Model file for the job. Use its own axes, mm. A direction names the side the tool comes from. Coordinates: 2 decimals unless noted, no trailing zeros. Order: outer loops, then holes, each group sorted by start corner. A loop starts at its lowest first (then second) coordinate and runs counter-clockwise, first axis right, second up. Notation, with made-up numbers: (62, 3.5) -> (94, 3.5) arc R18 cw to (94, 30.5) -> close; hole circle Ø1 at (-1, 13). An arc over 180 degrees is marked (long way). Return JSON: item names as keys, results as strings. Group by question number.
1) Probe line 1 (Y direction, x = -23.5, z = 47); line 2 (X direction, y = -41, z = 18); line 3 (Z direction, x = -39, y = -30.5). List the from-to ranges inside material, lowest first.
2) Cut at A-A (z = 11). Write the cut outline in (x, y), and give its area (3 significant figures).
3) Flat gauge pins, fed straight in: pin 1 (8 mm diameter, centred on y = -40.5, z = 21.5, fed in from +X); pin 2 (1 mm diameter, centred on y = -41.5, z = 12.5, fed in from -X). Where does each tip first touch, or does it go through?
4) Cut at B-B (x = -24.5). Write the cut outline in (y, z).
5) Which spindle directions (+Z, -Z, +X, -X, +Y, -Y) get a long thin tool onto all of the face, cutting with end or side? Do faces 1 (the flat face through (-25.588, -38, 14)), 2 (the flat face through (-43.156, -38, 14)), 3 (the flat face through (-32, -19, 0)). Say none if no direction does.
6) Cut at C-C (y = -45). Write the cut outline in (x, z), and give its area (3 significant figures).
7) Cut at D-D (x = -28.5). Write the cut outline in (y, z), and give its area (3 significant figures).
from build123d import *

# Parameters (mm, degrees)
F0_W     = 39.718569
F0_H     = 51.366802
F1_DEPTH = 25.4
F3_DEPTH = 25.4


with BuildPart() as f1:
    # F0 (on Front) → F1 (new body)
    with BuildSketch(Plane.XZ):
        with Locations((-31.316563, 25.683401)):
            Rectangle(F0_W, F0_H)
    extrude(amount=F1_DEPTH)

    # F2 (on face) → F3 (join)
    with BuildSketch(Plane.XZ.offset(25.4)):
        Polygon((-25.587924, 27.87938), (-43.155752, 28.070334), (-43.155752, 0), (-25.587924, 0), align=None)
    extrude(amount=F3_DEPTH)


solid = f1.part
Answers below:
{
 "1": {"line 1": "y = -25.4 to 0", "line 2": "x = -43.16 to -25.59", "line 3": "z = 0 to 28.03"},
 "2": {"outline": "(-51.18, -25.4) -> (-43.16, -25.4) -> (-43.16, -50.8) -> (-25.59, -50.8) -> (-25.59, -25.4) -> (-11.46, -25.4) -> (-11.46, 0) -> (-51.18, 0) -> close", "area": "1,460 mm^2"},
 "3": {"pin 1": "stops at x = -25.59", "pin 2": "stops at x = -43.16"},
 "4": {"outline": "(-25.4, 0) -> (0, 0) -> (0, 51.37) -> (-25.4, 51.37) -> close"},
 "5": {"face 1": "+Z, -Z, +X, -Y", "face 2": "+Z, -Z, -X, -Y", "face 3": "-Z, +X, -X, +Y, -Y"},
 "6": {"outline": "(-43.16, 0) -> (-25.59, 0) -> (-25.59, 27.88) -> (-43.16, 28.07) -> close", "area": "491 mm^2"},
 "7": {"outline": "(-50.8, 0) -> (0, 0) -> (0, 51.37) -> (-25.4, 51.37) -> (-25.4, 27.91) -> (-50.8, 27.91) -> close", "area": "2,010 mm^2"}
}
